Model file for the job. Use its own axes, mm. Face numbers are marked on the shaded views. A direction names the side the tool comes from. Round coordinates to 2 decimals unless told otherwise and drop trailing zeros. Loops run counter-clockwise (first coordinate to the right, second up) from the corner with the lowest first, then second, coordinate; pieces in that order, holes last. Notation, with made-up numbers: (48, 5) -> (90, 5) arc R27 cw to (90, 25) -> close; hole circle Ø1 at (-23.5, -32). An arc over 180 degrees is marked (long way). Use a Markdown table: item, result.
Autodesk Fusion 360 part; units mm, degrees
sketch "Platform" plane through (0, 0, 0) normal (0, 1, 0) x (1, 0, 0)
  line L0 (35, -68) -> (35, -60)
  line L1 (0, -76) -> (0, -68)
  line L2 (0, -68) -> (35, -68)
  line L3 (35, -60) -> (0, -60)
  line L4 (35, -76) -> (0, -76)
  line L5 (0, -60) -> (0, -68)
  line L6 (35, -68) -> (35, -76)
  line L7 (0, -68) -> (35, -68)
  dimension "d1" = 8
  dimension "d2" = 35
  dimension "d3" = 60
  dimension "d4" = 8
extrude "Extrude1" add sketch "Platform" along normal mid plane 35 contours L1 L2 L4 L6 L7
sketch "Puzzle" plane through (0, 0, 68) normal (0, 0, -1) x (-1, 0, 0)
  line L0 (0, -17.5) -> (0, 17.5)
  line L1 (0, 17.5) -> (-35, 17.5)
  line L2 (-35, 17.5) -> (-35, -17.5)
  line L3 (-35, -17.5) -> (0, -17.5)
  circle A0 centre (-3, 8.75) radius 5.2
  line L4 (0, -17.5) -> (-35, 0) construction
  line L5 (-17.5, -17.5) -> (-17.5, 0) construction
  line L6 (0, -17.5) -> (0, 17.5)
  circle A1 centre (3, 8.75) radius 5 construction
  line L7 (-32, -13.95) -> (-32, -3.55) construction
  circle A2 centre (-32, -8.75) radius 5.2
  circle A3 centre (-32, 8.75) radius 5.2 construction
  circle A4 centre (-32, -8.75) radius 5 construction
  line L8 (0, 0) -> (-35, 0) construction
  line L9 (0, 0) -> (-35, -17.5) construction
  circle A5 centre (-38, 8.75) radius 5
  line L10 (0, 17.5) -> (-35, 17.5)
  circle A6 centre (3, -8.75) radius 5
  line L11 (3, -13.75) -> (3, -3.75) construction
  line L12 (-35, -17.5) -> (0, -17.5)
  line L13 (-35, 17.5) -> (-35, -17.5)
  point P0 (-17.5, -8.75)
  dimension "d11" = 10
  dimension "d12" = 3
  dimension "d13" = 3
  dimension "d14" = 0.2
sketch "Adapter" plane through (0, 0, 68) normal (0, 0, -1) x (-1, 0, 0)
  line L0 (-35, 17.5) -> (-35, -17.5)
  line L1 (-35, -17.5) -> (0, -17.5)
  line L2 (0, -17.5) -> (0, 17.5)
  line L3 (0, 17.5) -> (-35, 17.5)
  circle A0 centre (-17.5, -9) radius 3
  circle A1 centre (-17.5, 9) radius 3
  line L4 (0, -6) -> (-35, -6) construction
  circle A2 centre (-17.5, 9) radius 3.2
  line L5 (0, 0) -> (-35, 0) construction
  circle A3 centre (-17.5, -9) radius 3.2
  line L6 (-35, -17.5) -> (0, 0) construction
  line L7 (0, -17.5) -> (-35, 0) construction
  line L8 (-17.5, -8.75) -> (-17.5, 0) construction
  point P0 (-17.5, 0)
  dimension "d26" = 6
  dimension "d27" = 0.2
  dimension "d28" = 6
extrude "Extrude6" cut sketch "Adapter" against normal blind 6 contours A0 | A1 | A2 | A3
chamfer "Chamfer1" distance 1.2 angle 45 2 edges at (20.4834, 10.1572, 74) (20.4834, -7.8428, 74)
extrude "PuzzleHoleLeft" cut sketch "Puzzle" against normal up to surface (8 mm away) contours L0 A0 L6 picked at (0.9006, 8.8366)
extrude "PuzzleHoleRight" [suppressed]
extrude "PuzzleStumpLeft" add sketch "Puzzle" against normal up to surface (8 mm away) contours L0 L6 A6 picked at (2.5946, -9.2349)
extrude "PuzzleStumpRight" [suppressed]
equation "d1 = PlatformHeight"
equation "d2 = LetterWidth"
equation "d3 = AdapterOffset"
equation "d4 = AdapterHeight"
equation "AdapterOffset = 60 mm"
equation "AdapterHeight = 8 mm"
equation "PlatformHeight = 8 mm"
equation "LetterWidth = 35 mm"
equation "d9 = LetterWidth"
equation "d11 = PuzzleRadius"
equation "d12 = PuzzleOffset"
equation "d13 = PuzzleOffset"
equation "d14 = Gap"
equation "PuzzleOffset = 3 mm"
equation "PuzzleRadius = 10 mm"
equation "Gap = 0.2 mm"
equation "d26 = AdapterHoleRadius"
equation "d27 = Gap"
equation "d28 = AdapterHoleSpread"
equation "AdapterHoleSpread = 6 mm"
equation "AdapterHoleRadius = 6 mm"
equation "AdapterHoleDepth = 6 mm"
equation "AdapterHoleBevel = 1.2 mm"
equation "d35 = AdapterHoleBevel"
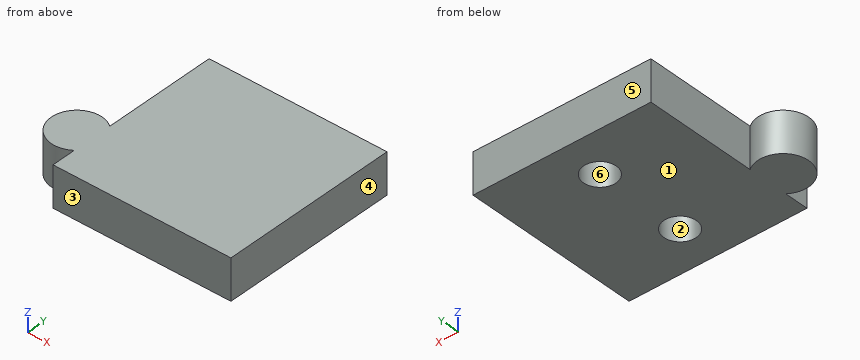
Q1. Band-saw the part on B-B, the plane y = 9. Give the cut face in (x, z).
Results list:
| item | result |
|---|---|
| outline | (0, 68) -> (14.3, 68) -> (14.3, 72.8) -> (15.5, 74) -> (19.5, 74) -> (20.7, 72.8) -> (20.7, 68) -> (35, 68) -> (35, 76) -> (0, 76) -> close |
Q2. Band-saw the part on D-D, the plane y = 2.5. Give the cut face in (x, z).
Results list:
| item | result |
|---|---|
| outline | (0, 68) -> (35, 68) -> (35, 76) -> (0, 76) -> close |
Q3. Tool access for the marked faces 1 and 2: list every direction of +Z, -Z, +X, -X, +Y, -Y with a clear straight run to the whole face (end or side of a thin tool).
Results list:
| item | result |
|---|---|
| face 1 | -Z, +X, -X, +Y, -Y |
| face 2 | -Z |
Q4. Flat gauge pins, fed straight in: pin 1 (4 mm diameter, centred on y = 10.5, z = 73, fed in from -X); pin 2 (2 mm diameter, centred on x = 18.5, y = 9.5, fed in from -Z); pin 3 (4.5 mm diameter, centred on x = 17.5, y = -9.5, fed in from -Z). Where does each tip first touch, or does it go through?
Results list:
| item | result |
|---|---|
| pin 1 | stops at x = 0 |
| pin 2 | stops at z = 73.88 |
| pin 3 | stops at z = 73.25 |
Q5. Band-saw the part on C-C, the plane x = -3. Give the cut face in (y, z).
Results list:
| item | result |
|---|---|
| outline | (-13.75, 68) -> (-3.75, 68) -> (-3.75, 76) -> (-13.75, 76) -> close |
Q6. Pull direction Y, two halves, no side cores. Call the marked faces 3, 4, 5 and 6: released by +Y, released by -Y, zero draft, split by the parting line, or undercut.
Results list:
| item | result |
|---|---|
| face 3 | released by -Y |
| face 4 | zero draft |
| face 5 | released by +Y |
| face 6 | undercut |
Q7. Drill centre lines: L1, parallel to Y at x = 17.5, z = 70.2; L2, parallel to X at y = -1, z = 74; L3, parallel to X at y = 8, z = 71.75. Where is each one in solid material? Low to high. Write a range as from..to.
Results list:
| item | result |
|---|---|
| L1 | y = -17.5..-12.2, -5.8..5.8, 12.2..17.5 |
| L2 | x = 0..35 |
| L3 | x = 0..14.46, 20.54..35 |
Q8. Band-saw the part on A-A, the plane z = 69. Give the cut face in (x, y).
Results list:
| item | result |
|---|---|
| outline | (0, -17.5) -> (35, -17.5) -> (35, 17.5) -> (0, 17.5) -> (0, -4.75) arc R5 ccw (long way) to (0, -12.75) -> close; hole circle Ø6.4 at (17.5, -9); hole circle Ø6.4 at (17.5, 9) |
